from build123d import *

# Parameters (mm, degrees)
MODEL_R             = 3.96875
MODEL_R_2           = 3.175
MODEL_R_3           = 4.1275
BOSS_EXTRUDE1_DEPTH = 19.05
CUT_EXTRUDE1_REACH  = 492.168
SKETCH2_R           = 2.5527
CUT_EXTRUDE2_REACH  = 492.168
SKETCH3_R           = 2.5527


with BuildPart() as part:
    # Model → Boss-Extrude1 (new body)
    with BuildSketch(Plane.XY):
        with BuildLine():
            Line((414.246385051, 270.805422424), (426.946385051, 270.805422424))
            ThreePointArc((426.946385051, 270.805422424), (435.926641172, 274.525166302), (439.646385051, 283.505422424))
            Line((439.646385051, 283.505422424), (439.646385051, 308.905422424))
            ThreePointArc((439.646385051, 308.905422424), (435.926641172, 317.885678545), (426.946385051, 321.605422424))
            Line((426.946385051, 321.605422424), (134.846385051, 321.605422424))
            ThreePointArc((134.846385051, 321.605422424), (125.86612893, 317.885678545), (122.146385051, 308.905422424))
            Line((122.146385051, 308.905422424), (122.146385051, 283.505422424))
            ThreePointArc((122.146385051, 283.505422424), (125.86612893, 274.525166302), (134.846385051, 270.805422424))
            Line((134.846385051, 270.805422424), (172.946385051, 270.805422424))
            ThreePointArc((172.946385051, 270.805422424), (217.847665656, 252.206703029), (236.446385051, 207.305422424))
            Line((236.446385051, 207.305422424), (236.446385051, 194.605422424))
            ThreePointArc((236.446385051, 194.605422424), (225.287153414, 167.66465406), (198.346385051, 156.505422424))
            Line((198.346385051, 156.505422424), (185.646385051, 156.505422424))
            ThreePointArc((185.646385051, 156.505422424), (176.66612893, 152.785678545), (172.946385051, 143.805422424))
            Line((172.946385051, 143.805422424), (172.946385051, 118.405422424))
            ThreePointArc((172.946385051, 118.405422424), (176.66612893, 109.425166302), (185.646385051, 105.705422424))
            Line((185.646385051, 105.705422424), (426.946385051, 105.705422424))
            ThreePointArc((426.946385051, 105.705422424), (435.926641172, 109.425166302), (439.646385051, 118.405422424))
            Line((439.646385051, 118.405422424), (439.646385051, 143.805422424))
            ThreePointArc((439.646385051, 143.805422424), (435.926641172, 152.785678545), (426.946385051, 156.505422424))
            Line((426.946385051, 156.505422424), (414.246385051, 156.505422424))
            ThreePointArc((414.246385051, 156.505422424), (387.305616688, 167.66465406), (376.146385051, 194.605422424))
            Line((376.146385051, 194.605422424), (376.146385051, 232.705422424))
            ThreePointArc((376.146385051, 232.705422424), (387.305616688, 259.646190787), (414.246385051, 270.805422424))
        make_face()
        with Locations(Location((357.096385051, 143.805422424, 0), (0, 0, 180))):
            Circle(MODEL_R, mode=Mode.SUBTRACT)
        with Locations(Location((357.096385051, 220.005422424, 0), (0, 0, 180))):
            Circle(MODEL_R, mode=Mode.SUBTRACT)
        with Locations(Location((357.096385051, 181.905422424, 0), (0, 0, 180))):
            Circle(MODEL_R, mode=Mode.SUBTRACT)
        with Locations(Location((395.196385051, 296.205422424, 0), (0, 0, 180))):
            Circle(MODEL_R_2, mode=Mode.SUBTRACT)
        with Locations(Location((357.096385051, 258.105422424, 0), (0, 0, 180))):
            Circle(MODEL_R, mode=Mode.SUBTRACT)
        with Locations(Location((357.096385051, 296.205422424, 0), (0, 0, 180))):
            Circle(MODEL_R, mode=Mode.SUBTRACT)
        with Locations(Location((271.371385051, 296.205422424, 0), (0, 0, 180))):
            Circle(MODEL_R_3, mode=Mode.SUBTRACT)
        with Locations(Location((318.996385051, 296.205422424, 0), (0, 0, 180))):
            Circle(MODEL_R, mode=Mode.SUBTRACT)
        with Locations(Location((318.996385051, 258.105422424, 0), (0, 0, 180))):
            Circle(MODEL_R, mode=Mode.SUBTRACT)
        with Locations(Location((166.596385051, 296.205422424, 0), (0, 0, 180))):
            Circle(MODEL_R_2, mode=Mode.SUBTRACT)
        with Locations(Location((318.996385051, 181.905422424, 0), (0, 0, 180))):
            Circle(MODEL_R, mode=Mode.SUBTRACT)
        with Locations(Location((395.196385051, 131.105422424, 0), (0, 0, 180))):
            Circle(MODEL_R_2, mode=Mode.SUBTRACT)
        with Locations(Location((318.996385051, 220.005422424, 0), (0, 0, 180))):
            Circle(MODEL_R, mode=Mode.SUBTRACT)
        with Locations(Location((318.996385051, 143.805422424, 0), (0, 0, 180))):
            Circle(MODEL_R, mode=Mode.SUBTRACT)
        with Locations(Location((217.396385051, 131.105422424, 0), (0, 0, 180))):
            Circle(MODEL_R_2, mode=Mode.SUBTRACT)
        with BuildLine():
            ThreePointArc((197.516747869, 136.500214247), (196.806510051, 131.105422424), (197.516747869, 125.7106306))
            ThreePointArc((197.516747869, 125.7106306), (194.115475863, 119.819454675), (188.224299938, 123.220726681))
            ThreePointArc((188.224299938, 123.220726681), (187.186260051, 131.105422424), (188.224299938, 138.990118166))
            ThreePointArc((188.224299938, 138.990118166), (194.115475863, 142.391390172), (197.516747869, 136.500214247))
        make_face(mode=Mode.SUBTRACT)
        with BuildLine():
            ThreePointArc((424.368470164, 123.220726681), (425.406510051, 131.105422424), (424.368470164, 138.990118166))
            ThreePointArc((424.368470164, 138.990118166), (418.477294239, 142.391390172), (415.076022233, 136.500214247))
            ThreePointArc((415.076022233, 136.500214247), (415.786260051, 131.105422424), (415.076022233, 125.7106306))
            ThreePointArc((415.076022233, 125.7106306), (418.477294239, 119.819454675), (424.368470164, 123.220726681))
        make_face(mode=Mode.SUBTRACT)
        with BuildLine():
            ThreePointArc((137.424299938, 304.090118166), (136.386260051, 296.205422424), (137.424299938, 288.320726681))
            ThreePointArc((137.424299938, 288.320726681), (143.315475863, 284.919454675), (146.716747869, 290.8106306))
            ThreePointArc((146.716747869, 290.8106306), (146.006510051, 296.205422424), (146.716747869, 301.600214247))
            ThreePointArc((146.716747869, 301.600214247), (143.315475863, 307.491390172), (137.424299938, 304.090118166))
        make_face(mode=Mode.SUBTRACT)
        with BuildLine():
            ThreePointArc((415.076022233, 290.8106306), (415.786260051, 296.205422424), (415.076022233, 301.600214247))
            ThreePointArc((415.076022233, 301.600214247), (418.477294239, 307.491390172), (424.368470164, 304.090118166))
            ThreePointArc((424.368470164, 304.090118166), (425.406510051, 296.205422424), (424.368470164, 288.320726681))
            ThreePointArc((424.368470164, 288.320726681), (418.477294239, 284.919454675), (415.076022233, 290.8106306))
        make_face(mode=Mode.SUBTRACT)
    extrude(amount=BOSS_EXTRUDE1_DEPTH)

    # Sketch2 → Cut-Extrude1 (cut, up to next)
    with BuildSketch(Plane.XZ.offset(-105.705422424), mode=Mode.PRIVATE) as cut_extrude1_sk1:
        with Locations((192.377385051, 9.525)):
            Circle(SKETCH2_R)
    cut_extrude1_tool1 = extrude(cut_extrude1_sk1.sketch, amount=-CUT_EXTRUDE1_REACH, mode=Mode.PRIVATE) & part.part
    # Sketch2 → Cut-Extrude1 (cut, up to next)
    with BuildSketch(Plane.XZ.offset(-105.705422424), mode=Mode.PRIVATE) as cut_extrude1_sk2:
        with Locations((420.215385051, 9.525)):
            Circle(SKETCH2_R)
    cut_extrude1_tool2 = extrude(cut_extrude1_sk2.sketch, amount=-CUT_EXTRUDE1_REACH, mode=Mode.PRIVATE) & part.part
    add(cut_extrude1_tool1.solids().sort_by_distance((192.377385, 105.705422, 9.525))[0], mode=Mode.SUBTRACT)
    add(cut_extrude1_tool2.solids().sort_by_distance((420.215385, 105.705422, 9.525))[0], mode=Mode.SUBTRACT)

    # Sketch3 → Cut-Extrude2 (cut, up to next)
    with BuildSketch(Plane(origin=(0, 321.605422424, 0), x_dir=(1, 0, 0), z_dir=(0, 1, 0)), mode=Mode.PRIVATE) as cut_extrude2_sk1:
        with Locations(Location((141.577385051, -9.525, 0), (0, 0, 180))):
            Circle(SKETCH3_R)
    cut_extrude2_tool1 = extrude(cut_extrude2_sk1.sketch, amount=-CUT_EXTRUDE2_REACH, mode=Mode.PRIVATE) & part.part
    # Sketch3 → Cut-Extrude2 (cut, up to next)
    with BuildSketch(Plane(origin=(0, 321.605422424, 0), x_dir=(1, 0, 0), z_dir=(0, 1, 0)), mode=Mode.PRIVATE) as cut_extrude2_sk2:
        with Locations((420.215385051, -9.525)):
            Circle(SKETCH3_R)
    cut_extrude2_tool2 = extrude(cut_extrude2_sk2.sketch, amount=-CUT_EXTRUDE2_REACH, mode=Mode.PRIVATE) & part.part
    add(cut_extrude2_tool1.solids().sort_by_distance((141.577385, 321.605422, 9.525))[0], mode=Mode.SUBTRACT)
    add(cut_extrude2_tool2.solids().sort_by_distance((420.215385, 321.605422, 9.525))[0], mode=Mode.SUBTRACT)


solid = part.part
Geometry: final body of the model. Coordinates: model frame, mm. A direction names the side the tool comes from. Coordinates: 2 decimals unless noted, no trailing zeros. Loops run counter-clockwise (first coordinate to the right, second up) from the corner with the lowest first, then second, coordinate; pieces in that order, holes last. Notation, with made-up numbers: (45.5, 1) - (101.5, 1) arc R22 ccw to (101.5, 8) - close; hole circle Ø1 at (-9, 41.25). An arc over 180 degrees is marked (long way). Put each result on its own line as item: value. Start each with the question number.
Q1. Line query: line 1 (X direction, y = 130.5, z = 9.75); line 2 (X direction, y = 305, z = 10.25); line 3 (X direction, y = 131, z = 10.5). Output: solid intervals per line, ascending.
Q2. Pin query (flat end, axial travel): pin 1 Ø6 at (x, z) = (420.22, 9.52) entering from -Y; pin 2 Ø8 at (y, z) = (261, 13.5) entering from +X; pin 3 Ø3 at (x, z) = (420.22, 9.52) entering from +Y; pin 4 Ø3 at (x, z) = (192.38, 9.52) entering from -Y. Return the tip coordinate at first contact, or that it passes through.
Q3. Cut plane A-A, the plane y = 164. Return loops of the section in (x, z), and give its area (3 significant figures).
Q4. Cut plane B-B, the plane z = 15. Give the number of separate pieces and of enclosed holes in the cut face, and give its area (3 significant figures).
Q5. Pull-direction query (X, two-part tool) for faces 1 (the cylindrical face through (194.01, 142.42, 9.39)), 2 (the cylindrical face through (225.58, 167.96, 9.39)), 3 (the flat face through (439.646, 296, 9)), 4 (the flat face through (305, 105.705, 9)); classes: released by +X, released by -X, zero draft, split by the parting line, or undercut.
Q6. Set-up query: faces 5 (the flat face through (279, 215, 19.05)), 6 (the flat face through (172.946, 131, 9)), 7 (the cylindrical face through (217.35, 252.7, 9.39)), 8 (the cylindrical face through (425.406, 130.994, 9.392)). Return all of +Z, -Z, +X, -X, +Y, -Y with unobstructed straight access to the full face (end or side cutting, diameter ignored); none if empty.
Q7. Cut plane C-C, the plane y = 245. Return loops of the section in (x, z), and give its area (3 significant figures).
Filled sheet:
1. line 1: 172.95 to 187.19, 196.82 to 214.28, 220.51 to 392.08, 398.31 to 415.78, 425.4 to 439.65
1. line 2: 122.15 to 137.77, 146.37 to 415.42, 424.02 to 439.65
1. line 3: 172.95 to 187.19, 196.81 to 214.22, 220.57 to 392.02, 398.37 to 415.79, 425.41 to 439.65
2. pin 1: y = 105.71
2. pin 2: x = 394.03
2. pin 3: y = 285.19
2. pin 4: y = 142.12
3. outline: (221.04, 0) - (391.55, 0) - (391.55, 19.05) - (221.04, 19.05) - close
3. area: 3,250 mm²
4. separate pieces: 1
4. enclosed holes: 19
4. area: 45,700 mm²
5. face 1: undercut
5. face 2: released by -X
5. face 3: released by +X
5. face 4: zero draft
6. face 5: +Z, +X, -X, +Y, -Y
6. face 6: +Z, -Z, -X, -Y
6. face 7: +Z, -Z, -X
6. face 8: +Z, -Z
7. outline: (224.05, 0) - (378.18, 0) - (378.18, 19.05) - (224.05, 19.05) - close
7. area: 2,940 mm²
